Verification items for the finished model (mm, model axes). Coordinates: 2 decimals unless noted, no trailing zeros. Order: outer loops, then holes, each group sorted by start corner. A loop starts at its lowest first (then second) coordinate and runs counter-clockwise, first axis right, second up. Notation, with made-up numbers: M -20,-20 L -16,-20 A31 ccw -16,13 Z; hole C 27,-6.5 d10. An arc over 180 degrees is marked long. Answer as a JSON object with one key per item and string values. Group by question number.
(1) Material ranges on line 1 (Y direction, x = 0, z = 15.5); line 2 (X direction, y = 76.5, z = 16.75); line 3 (X direction, y = 66, z = 3.5), recorded low to high.
(2) Gauge pin test, flat ends, axial feed: pin 1 Ø1.5 at (x, z) = (5, 7.5) entering from -Y; pin 2 Ø5 at (x, z) = (15.5, 17) entering from +Y. Record the tip position at first contact, or that the pin passes through.
(3) Cross-section at C-C (z = 13). Enter the section's corners in (x, y).
(4) Cross-section at B-B (y = 69.5). Enter the section's corners in (x, z).
(5) Cross-section at A-A (x = 0). Enter the section's corners in (y, z).
(6) Mould release check, pull along X, two halves, no side actions. Record for faces 1 (the face through (-2.75, 63.8, 12.88)), 2 (the face through (0, 40, 0)), 3 (the face through (25.4, 38, 13)), 4 (the face through (-25.4, 39, 13)): released by +X, released by -X, zero draft, split by the parting line, or undercut.
(7) Cross-section at D-D (x = 16). Enter the section's corners in (y, z).
from build123d import *

# Parameters (mm, degrees)
F1_DEPTH = 25.4
F2_R     = 12.7
F3_DEPTH = 25.4


with BuildPart() as f1:
    # F0 (on Top) → F1 (new body)
    with BuildSketch(Plane.XY):
        with BuildLine():
            Line((-25.4, 76.2), (-25.4, 0))
            Line((-25.4, 0), (25.4, 0))
            Line((25.4, 0), (25.4, 76.2))
            ThreePointArc((25.4, 76.2), (0, 50.8), (-25.4, 76.2))
        make_face()
        with BuildLine():
            ThreePointArc((25.4, 76.2), (0, 101.6), (-25.4, 76.2))
            Line((-25.4, 76.2), (25.4, 76.2))
        make_face()
        with BuildLine():
            Line((25.4, 76.2), (-25.4, 76.2))
            ThreePointArc((-25.4, 76.2), (0, 50.8), (25.4, 76.2))
        make_face()
    extrude(amount=F1_DEPTH)

    # F2 (on face) → F3 (cut)
    with BuildSketch(Plane.XY.offset(25.4)):
        with Locations((0, 76.2)):
            Circle(F2_R)
    extrude(amount=-F3_DEPTH, mode=Mode.SUBTRACT)


solid = f1.part
Taken from the geometry:
{
 "1": {"line 1": "y = 0 to 63.5, 88.9 to 101.6", "line 2": "x = -25.4 to -12.7, 12.7 to 25.4", "line 3": "x = -25.4 to -7.57, 7.57 to 25.4"},
 "2": {"pin 1": "stops at y = 0", "pin 2": "stops at y = 98.02"},
 "3": {"outline": "M -25.4,0 L 25.4,0 L 25.4,76.2 A25.4 ccw -25.4,76.2 Z; hole C 0,76.2 d25.4"},
 "4": {"outline": "M -25.4,0 L -10.79,0 L -10.79,25.4 L -25.4,25.4 Z; M 10.79,0 L 25.4,0 L 25.4,25.4 L 10.79,25.4 Z"},
 "5": {"outline": "M 0,0 L 63.5,0 L 63.5,25.4 L 0,25.4 Z; M 88.9,0 L 101.6,0 L 101.6,25.4 L 88.9,25.4 Z"},
 "6": {"face 1": "undercut", "face 2": "zero draft", "face 3": "released by +X", "face 4": "released by -X"},
 "7": {"outline": "M 0,0 L 95.93,0 L 95.93,25.4 L 0,25.4 Z"}
}
